Autodesk Inventor part; units mm, degrees
ref_plane "YZ Plane" through (0, 0, 0) normal (1, 0, 0) x (0, 1, 0)
ref_plane "XZ Plane" through (0, 0, 0) normal (0, 1, 0) x (-1, 0, 0)
ref_plane "XY Plane" through (0, 0, 0) normal (0, 0, 1) x (1, 0, 0)
sketch "Sketch2" plane through (0, 0, 0) normal (0, 0, 1) x (1, 0, 0)
  line L0 (-8.2799, 8.6846) -> (-1.9299, 8.6846)
  line L1 (-1.9299, 8.6846) -> (-1.9299, -4.0154)
  line L2 (-1.9299, -4.0154) -> (-8.2799, -4.0154)
  line L3 (-8.2799, -4.0154) -> (-8.2799, 8.6846)
  point P0 (0, 0)
  dimension "d3" = 6.35
  dimension "d5" = 12.7
extrude "Extrusion1" add sketch "Sketch2" along normal blind 228.6
sketch "Sketch3" plane through (-1.9299, -4.0154, 0) normal (1, 0, 0) x (0, 0, -1)
  point P0 (-228.6, 12.7)
  point P1 (0, 4.0154)
  point P2 (-210.82, 9.287)
  point P3 (-30.6578, 9.6266)
  dimension "d8" = 3.413
  dimension "d9" = 17.78
  dimension "d45" = 197.9422
  dimension "d46" = 3.0734
hole "Hole1" at (-1.9299, 5.2716, 210.82) direction (-1, 0, 0) diameter 1.7018 end through all
pattern_linear "Rectangular Pattern1" count 7 spacing 25.4 along (0, 0, -1) of "Hole1"
sketch "Sketch6" plane through (203.1751, -4.0154, 104.775) normal (0, -1, 0) x (1, 0, 0)
  point P0 (0, 4.0154)
  point P1 (-208.28, -100.965)
  point P2 (-208.28, -46.355)
  point P3 (-211.455, -104.775)
  point P4 (-205.105, -104.775)
  dimension "d68" = 58.42
  dimension "d69" = 3.81
  dimension "d76" = 3.175
  dimension "d77" = 3.175
hole "Hole2" at (-5.1049, -4.0154, 3.81) direction (0, 1, 0) diameter 1.7018 depth 6.35 tip angle 118
hole "Hole5" at (-5.1049, -4.0154, 58.42) direction (0, 1, 0) diameter 1.7018 depth 6.35 tip angle 118
pattern_linear "Rectangular Pattern5" count 2 spacing 25.4 along (0, 0, 1) of "Hole2"
pattern_linear "Rectangular Pattern6" count 5 spacing 38.1 along (0, 0, 1) of "Hole5"
sketch "Sketch9" plane through (-8.2799, -4.0154, 0) normal (0, -1, 0) x (1, 0, 0)
  line L0 (6.35, 0) -> (6.35, 228.6)
  line L1 (0, 0) -> (0, 228.6)
  line L2 (6.35, 0) -> (0, 0)
  line L3 (0, 0) -> (6.35, 0)
  line L4 (6.35, 30.6578) -> (0, 30.6578) construction
  line L5 (6.096, 16.4084) -> (0, 16.4084) construction
  line L6 (0, 0) -> (0, 228.6) construction
  line L7 (6.35, 2.159) -> (0, 2.159) construction
  line L8 (1.524, 32.6898) -> (0, 32.6898)
  line L9 (0, 32.6898) -> (0, 28.6258)
  line L10 (0, 28.6258) -> (1.524, 28.6258)
  line L11 (1.524, 28.6258) -> (1.524, 32.6898)
  line L12 (1.524, 32.6898) -> (0, 28.6258) construction
  line L13 (0, 32.6898) -> (1.524, 28.6258) construction
  line L14 (1.524, 18.4404) -> (0, 18.4404)
  line L15 (0, 18.4404) -> (0, 14.3764)
  line L16 (0, 14.3764) -> (1.524, 14.3764)
  line L17 (1.524, 14.3764) -> (1.524, 18.4404)
  line L18 (1.524, 18.4404) -> (0, 14.3764) construction
  line L19 (0, 18.4404) -> (1.524, 14.3764) construction
  line L20 (1.524, 4.318) -> (0, 4.318)
  line L21 (0, 4.318) -> (0, 0)
  line L22 (0, 0) -> (1.524, 0)
  line L23 (1.524, 0) -> (1.524, 4.318)
  line L24 (1.524, 4.318) -> (0, 0) construction
  line L25 (0, 4.318) -> (1.524, 0) construction
  point P0 (6.35, 4.191)
  point P1 (4.318, 0)
  point P2 (0.762, 30.6578)
  point P3 (0.762, 16.4084)
  point P4 (0.762, 2.159)
  dimension "d78" = 30.6578
  dimension "d93" = 4.064
  dimension "d94" = 1.524
  dimension "d95" = 1.524
  dimension "d96" = 4.064
  dimension "d97" = 1.524
extrude "Extrusion3" cut sketch "Sketch9" against normal through all
properties part number "mounting rail 9.0 x.250 x.500-A-sfpcutouts" material "Gold"
For this review, take the finished solid that the model builds, in its own axes (mm). A direction names the side the tool comes from. Coordinates: 2 decimals unless noted, no trailing zeros. Answer as CSV lines item,"result".
Q1. Draft analysis for pull direction Z (two halves, no side actions). For faces 4 (the face through (-5, 2, 228.6)), 5 (the face through (-6.756, 2, 16)), 6 (the face through (-8.28, 2, 9)), state which applies: released by +Z, released by -Z, zero draft, split by the parting line, or undercut.
Model answer:
face 4,"released by +Z"
face 5,"undercut"
face 6,"zero draft"
Q2. For faces 1 (the face through (-6.756, 2, 2)), 2 (the face through (-6.756, 2, 31)), 3 (the face through (-8.28, 2, 23)), list the 3-axis set-ups (+Z, -Z, +X, -X, +Y, -Y) from which the entire face can be reached by the end or side of a thin tool; tool diameter is ignored.
Model answer:
face 1,"-Z, -X, +Y, -Y"
face 2,"-X, +Y, -Y"
face 3,"+Z, -Z, -X, +Y, -Y"
Q3. Clearance check with flat-ended pins moving along their axes: pin 1 Ø0.8 at (x, y) = (-8, 2) entering from -Z; pin 2 Ø3.5 at (y, z) = (2, 1.5) entering from -X; pin 3 Ø1.5 at (y, z) = (5.27, 160.02) entering from +X (3 decimals). State where each tip first meets the part, or that it passes through.
Model answer:
pin 1,"stops at z = 4.32"
pin 2,"stops at x = -6.76"
pin 3,"passes through"
Q4. Wall thickness on line 1 along Z through (x, y) = (-7, 7); line 2 along Y through (x, z) = (-4, 185.42); line 3 along X through (y, z) = (-0.75, 172.72): over which ranges is each line inside the solid? List them lowest first. Write a range as [from, to].
Model answer:
line 1,"z = [4.32, 14.38], [18.44, 28.63], [32.69, 228.6]"
line 2,"y = [-4.02, 4.42], [6.12, 8.68]"
line 3,"x = [-8.28, -5.96], [-4.25, -1.93]"
